Geometry check sheet. Reference: the model listing, model coordinates, mm. A direction names the side the tool comes from. Round coordinates to 2 decimals unless told otherwise and drop trailing zeros. Loops run counter-clockwise (first coordinate to the right, second up) from the corner with the lowest first, then second, coordinate; pieces in that order, holes last. Notation, with made-up numbers: (76.25, 89) -> (135.25, 89) arc R23 cw to (135.25, 120) -> close; hole circle Ø10 at (-10, 80). An arc over 180 degrees is marked (long way). Use a Markdown table: item, result. Add a question column.
Q1. Set-up check for faces 4 (the face through (-3, 3, 0)), 5 (the face through (-7.493, -0.33, 14.367)): record each of +Z, -Z, +X, -X, +Y, -Y from which the full face is reachable in a straight line by a thin tool's end or side.
Q2. Gauge pin test, flat ends, axial feed: P1, Ø2, axis at x = -8.49, y = 8.49, coming from the +Z side; P2, Ø5, axis at x = -2.5, z = 21, coming from the -Y side; P3, Ø5.5, axis at x = 8.49, y = 8.49, coming from the +Z side; P4, Ø5, axis at x = -3, z = 14.5, coming from the +Y side. Record the tip position at first contact, or that the pin passes through.
Q3. Material ranges on L1, parallel to Y at x = 8, z = 2.5; L2, parallel to Y at x = -10, z = 3.25; L3, parallel to Y at x = 0.25, z = 15, recorded low to high.
Q4. Sectioned sample at C-C, the plane x = 8. Enter the section's corners in (y, z).
Q5. Release check for a two-part mould opening along X. For faces 1 (the face through (8.71, -6.75, 2.46)), 2 (the face through (-11, -12, 3)), 3 (the face through (11, -12, 2)) record: released by +X, released by -X, zero draft, split by the parting line, or undercut.
Q6. Sectioned sample at D-D, the plane z = 6. Enter the section's corners in (x, y).
Q7. Sectioned sample at A-A, the plane x = 0. Enter the section's corners in (y, z).
Autodesk Inventor part; units mm, degrees
ref_plane "YZ Plane" through (0, 0, 0) normal (1, 0, 0) x (0, 1, 0)
ref_plane "XZ Plane" through (0, 0, 0) normal (0, 1, 0) x (-1, 0, 0)
ref_plane "XY Plane" through (0, 0, 0) normal (0, 0, 1) x (1, 0, 0)
sketch "Sketch1" plane through (0, 0, 0) normal (0, 0, 1) x (1, 0, 0)
  line L0 (-12.5, 12.5) -> (12.5, 12.5)
  line L1 (12.5, 12.5) -> (12.5, -12.5)
  line L2 (12.5, -12.5) -> (-12.5, -12.5)
  line L3 (-12.5, -12.5) -> (-12.5, 12.5)
  line L4 (-12.5, 12.5) -> (12.5, -12.5) construction
  line L5 (12.5, 12.5) -> (-12.5, -12.5) construction
  point P0 (0, 0)
  dimension "d0" = 25
  dimension "d1" = 25
extrude "Extrusion1" add sketch "Sketch1" along normal blind 5
sketch "Sketch2" plane through (0, 0, 5) normal (0, 0, 1) x (1, 0, 0)
  circle A0 centre (0, 0) radius 7.5
  dimension "d4" = 15
extrude "Extrusion2" add sketch "Sketch2" along normal blind 19
sketch "Sketch3" plane through (0, 0, 24) normal (0, 0, 1) x (1, 0, 0)
  circle A0 centre (0, 0) radius 4
  dimension "d7" = 8
extrude "Extrusion3" cut sketch "Sketch3" against normal blind 30
sketch "Sketch4" plane through (0, 0, 0) normal (0, 0, -1) x (-1, 0, 0)
  circle A0 centre (0, 0) radius 12
  line L0 (-12.5, -12.5) -> (-12.5, 12.5)
  line L1 (12.5, 12.5) -> (12.5, -12.5)
  line L2 (-12.5, 12.5) -> (8.4853, -8.4853)
  circle A1 centre (8.4853, -8.4853) radius 1.75
  circle A2 centre (8.4853, 8.4853) radius 1.75
  circle A3 centre (-8.4853, 8.4853) radius 1.75
  circle A4 centre (-8.4853, -8.4853) radius 1.75
  dimension "d10" = 24
  dimension "d11" = 3.5
  dimension "d14" = 360
extrude "Extrusion4" cut sketch "Sketch4" against normal blind 30 contours A2 A0 | A0 A2 | A1 A0 | A0 L2 A1 | A0 A1 L2 | A3 L2 A0 | A0 L2 A3 | A3 A0 L2 | A0 A3 L2 | A4 A0 | A0 A4
chamfer "Chamfer1" distance 2 angle 45 4 edges at (12.5, 12.5, 2.5) (-12.5, 12.5, 2.5) (-12.5, -12.5, 2.5) (12.5, -12.5, 2.5)
properties part number "RODAMIENTO LINEAL"
Values:
| question | item | result |
|---|---|---|
| 1 | face 4 | -Z, +X, -X, +Y, -Y |
| 1 | face 5 | +Z |
| 2 | P1 | through |
| 2 | P2 | y = -7.5 |
| 2 | P3 | z = 5 |
| 2 | P4 | y = 7.48 |
| 3 | L1 | -12.5 to -10.17, -6.8 to 6.8, 10.17 to 12.5 |
| 3 | L2 | -12.5 to -9.36, -7.61 to 7.61, 9.36 to 12.5 |
| 3 | L3 | -7.5 to -3.99, 3.99 to 7.5 |
| 4 | outline | (-12.5, 0) -> (-10.17, 0) -> (-10.17, 5) -> (-12.5, 5) -> close; (-6.8, 0) -> (6.8, 0) -> (6.8, 5) -> (-6.8, 5) -> close; (10.17, 0) -> (12.5, 0) -> (12.5, 5) -> (10.17, 5) -> close |
| 5 | face 1 | undercut |
| 5 | face 2 | released by -X |
| 5 | face 3 | released by +X |
| 6 | outline | circle Ø15 at (0, 0); hole circle Ø8 at (0, 0) |
| 7 | outline | (-12.5, 0) -> (-4, 0) -> (-4, 24) -> (-7.5, 24) -> (-7.5, 5) -> (-12.5, 5) -> close; (4, 0) -> (12.5, 0) -> (12.5, 5) -> (7.5, 5) -> (7.5, 24) -> (4, 24) -> close |
